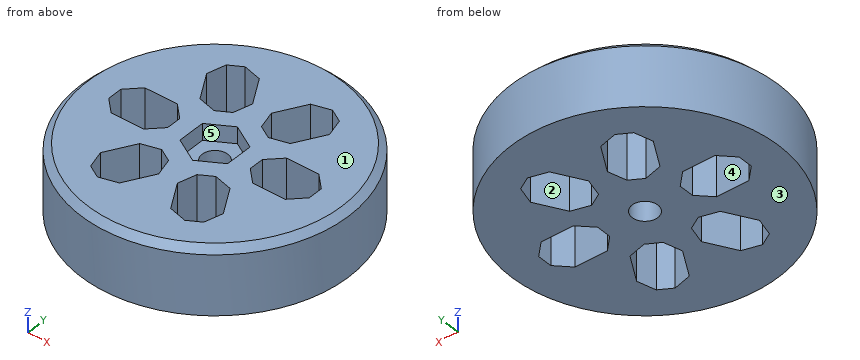
```python
from build123d import *

# Parameters (mm, degrees)
SKETCH1_R               = 25.6159
BOSS_EXTRUDE1_DEPTH     = 12.7
CHAMFER1_SIZE           = 1.27
CUT_EXTRUDE1_DEPTH      = 3.175
F_8_CLEARANCE_HOLE1_D   = 4.9149
SKETCH5_W               = 11.3284
SKETCH5_H               = 7.9375
CUT_EXTRUDE_THIN1_DEPTH = 13.7
CHAMFER2_SIZE           = 2.54


with BuildPart() as part:
    # Sketch1 → Boss-Extrude1 (new body)
    with BuildSketch(Plane.XY):
        Circle(SKETCH1_R)
    extrude(amount=BOSS_EXTRUDE1_DEPTH)

    # Chamfer1
    chamfer1_edges = [part.edges().sort_by_distance(p)[0] for p in [
        (-25.6159, 0, 12.7),
    ]]
    chamfer(chamfer1_edges, length=CHAMFER1_SIZE)

    # Sketch2 → Cut-Extrude1 (cut)
    with BuildSketch(Plane.XY.offset(12.7)):
        Polygon((-4.572, -2.639645431), (0, -5.279290861), (4.572, -2.639645431), (4.572, 2.639645431), (0, 5.279290861), (-4.572, 2.639645431), align=None)
    extrude(amount=-CUT_EXTRUDE1_DEPTH, mode=Mode.SUBTRACT)

    # #8 Clearance Hole1 (through all)
    with Locations(Plane.XY.offset(12.7)):
        with Locations((0, 0)):
            Hole(F_8_CLEARANCE_HOLE1_D / 2)

    # Sketch5 → Cut-Extrude-Thin1 (cut, through all)
    with BuildSketch(Plane.XY.offset(12.7)):
        Polygon((-7.405788321, -4.889701643), (-13.069988321, -14.700383827), (-6.195911679, -18.669133827), (-0.531711679, -8.858451643), align=None)
        with Locations((-13.6017, 0)):
            Rectangle(SKETCH5_W, SKETCH5_H)
        Polygon((-0.531711679, 8.858451643), (-6.195911679, 18.669133827), (-13.069988321, 14.700383827), (-7.405788321, 4.889701643), align=None)
        Polygon((7.405788321, 4.889701643), (13.069988321, 14.700383827), (6.195911679, 18.669133827), (0.531711679, 8.858451643), align=None)
        with Locations((13.6017, 0)):
            Rectangle(SKETCH5_W, SKETCH5_H)
        Polygon((0.531711679, -8.858451643), (6.195911679, -18.669133827), (13.069988321, -14.700383827), (7.405788321, -4.889701643), align=None)
    extrude(amount=-CUT_EXTRUDE_THIN1_DEPTH, mode=Mode.SUBTRACT)

    # Chamfer2
    chamfer2_edges = [part.edges().sort_by_distance(p)[0] for p in [
        (6.195911679, -18.669133827, 6.35),
        (0.531711679, -8.858451643, 6.35),
        (7.405788321, -4.889701643, 6.35),
        (13.069988321, -14.700383827, 6.35),
        (19.2659, -3.96875, 6.35),
        (7.9375, -3.96875, 6.35),
        (7.9375, 3.96875, 6.35),
        (19.2659, 3.96875, 6.35),
        (13.069988321, 14.700383827, 6.35),
        (7.405788321, 4.889701643, 6.35),
        (0.531711679, 8.858451643, 6.35),
        (6.195911679, 18.669133827, 6.35),
        (-6.195911679, 18.669133827, 6.35),
        (-0.531711679, 8.858451643, 6.35),
        (-7.405788321, 4.889701643, 6.35),
        (-13.069988321, 14.700383827, 6.35),
        (-19.2659, 3.96875, 6.35),
        (-7.9375, 3.96875, 6.35),
        (-7.9375, -3.96875, 6.35),
        (-19.2659, -3.96875, 6.35),
        (-13.069988321, -14.700383827, 6.35),
        (-7.405788321, -4.889701643, 6.35),
        (-0.531711679, -8.858451643, 6.35),
        (-6.195911679, -18.669133827, 6.35),
    ]]
    chamfer(chamfer2_edges, length=CHAMFER2_SIZE)


solid = part.part
```
Read the model definition and answer for the solid it produces. Units are mm, in the model's axes. Face numbers are marked on the shaded views. A direction names the side the tool comes from. Coordinates: 2 decimals unless noted, no trailing zeros. Order: outer loops, then holes, each group sorted by start corner. A loop starts at its lowest first (then second) coordinate and runs counter-clockwise, first axis right, second up. Notation, with made-up numbers: (39, 78.25) - (57, 78.25) arc R21 cw to (57, 98.25) - close; hole circle Ø10 at (41, 76.25). An arc over 180 degrees is marked (long way). Answer as a JSON object with one key per item and string values. Group by question number.
Item 1: Consider probe 1 along Y at (x, z) = (3, 9); probe 2 along Y at (x, z) = (0, 3.25); probe 3 along X at (y, z) = (-3, 3.25). Determine where each line is inside the solid, lowest interval first. Write a range as from..to.
Item 2: The mould has two halves that part along X. Classify the marked faces 1 and 2: +X half, -X half, draft (parallel to the pull), parting line (faces both ways), or undercut.
Item 3: Flat-ended cylindrical pins translate along their axes: P1, Ø6, axis at x = 20.5, z = 2, coming from the +Y side; P2, Ø2, axis at y = -14.5, z = 10, coming from the -X side; P3, Ø5, axis at x = 15, z = 4.5, coming from the -Y side. Find the tip coordinate at first contact, or state that the pin passes through.
Item 4: Section A-A (y = 0) is taken. Give the vertices of the cut face in (x, z) (1 decimal), plus the area to 3 significant figures.
Item 5: A tool of negligible diameter and unlimited length cuts with its end or side. For the marked faces 3, 4 and 5, from which of +Z, -Z, +X, -X, +Y, -Y can it reach the whole face along a straight path? Write none if from no direction.
Item 6: Section B-B (z = 7.25) is taken. State how many separate pieces and enclosed holes the cut face has, plus the area to 3 significant figures.
Results are:
{
 "1": {"probe 1": "y = -25.44..-13.13, -7.43..7.43, 13.13..25.44", "probe 2": "y = -25.62..-2.46, 2.46..25.62", "probe 3": "x = -25.44..-17.69, -9.51..9.51, 17.69..25.44"},
 "2": {"face 1": "draft", "face 2": "undercut"},
 "3": {"P1": "stops at y = 18.71", "P2": "stops at x = -21.77", "P3": "stops at y = -22.36"},
 "4": {"outline": "(-25.6, 0) - (-19.3, 0) - (-19.3, 12.7) - (-24.3, 12.7) - (-25.6, 11.4) - close; (-7.9, 0) - (-2.5, 0) - (-2.5, 9.5) - (-4.6, 9.5) - (-4.6, 12.7) - (-7.9, 12.7) - close; (2.5, 0) - (7.9, 0) - (7.9, 12.7) - (4.6, 12.7) - (4.6, 9.5) - (2.5, 9.5) - close; (19.3, 0) - (25.6, 0) - (25.6, 11.4) - (24.3, 12.7) - (19.3, 12.7) - close", "area": "285 mm^2"},
 "5": {"face 3": "-Z, +X, -X, +Y, -Y", "face 4": "+Z, -Z", "face 5": "+Z"},
 "6": {"separate pieces": "1", "enclosed holes": "7", "area": "1,580 mm^2"}
}
